Read the model definition and answer for the solid it produces. Units are mm, in the model's axes. Give positions to 0.01 mm unless a question says otherwise; leave off trailing zeros. Loops run counter-clockwise (first coordinate to the right, second up) from the corner with the lowest first, then second, coordinate; pieces in that order, holes last. Notation, with made-up numbers: (-32, -15) - (15, -15) arc R11 ccw to (15, 3) - close; hole circle Ø4 at (-8, 41). An arc over 180 degrees is marked (long way). Write item = value, one per line.
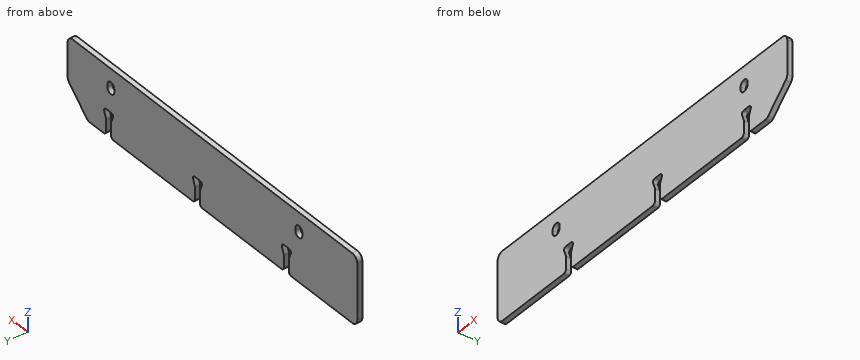
```python
from build123d import *

# Parameters (mm, degrees)
SKETCH2_W           = 114
SKETCH2_H           = 21.5
BOSS_EXTRUDE1_DEPTH = 1.5875
CHAMFER1_SIZE       = 8
FILLET1_R           = 2
CUT_EXTRUDE1_DEPTH  = 2.5875
LPATTERN1_COUNT     = 3
LPATTERN1_PITCH     = 35
FILLET2_R           = 1
FILLET3_R           = 1


with BuildPart() as part:
    # Sketch2 → Boss-Extrude1 (new body)
    with BuildSketch(Plane(origin=(0, 0, 0), x_dir=(1, 0, 0), z_dir=(0, 1, 0))):
        with Locations((-3, 10.75)):
            Rectangle(SKETCH2_W, SKETCH2_H)
        with BuildLine():
            Line((-38.35, 5.5), (-38.35, 6.5))
            ThreePointArc((-38.35, 6.5), (-37, 7.85), (-35.65, 6.5))
            Line((-35.65, 6.5), (-35.65, 5.5))
            ThreePointArc((-35.65, 5.5), (-37, 4.15), (-38.35, 5.5))
        make_face(mode=Mode.SUBTRACT)
        with BuildLine():
            Line((35.65, 5.5), (35.65, 6.5))
            ThreePointArc((35.65, 6.5), (37, 7.85), (38.35, 6.5))
            Line((38.35, 6.5), (38.35, 5.5))
            ThreePointArc((38.35, 5.5), (37, 4.15), (35.65, 5.5))
        make_face(mode=Mode.SUBTRACT)
    extrude(amount=BOSS_EXTRUDE1_DEPTH)

    # Chamfer1
    chamfer1_edges = [part.edges().sort_by_distance(p)[0] for p in [
        (54, 0.79375, -21.5),
    ]]
    chamfer(chamfer1_edges, length=CHAMFER1_SIZE)

    # Fillet1
    fillet1_edges = [part.edges().sort_by_distance(p)[0] for p in [
        (46, 0.79375, -21.5),
        (54, 0.79375, -13.5),
        (-60, 0.79375, 0),
        (-60, 0.79375, -21.5),
        (54, 0.79375, 0),
    ]]
    fillet(fillet1_edges, radius=FILLET1_R)

    # Sketch3 → Cut-Extrude1 (cut, through all)
    with BuildSketch(Plane(origin=(0, 0, 0), x_dir=(1, 0, 0), z_dir=(0, 1, 0))):
        with BuildLine():
            Line((-33.075, 21.5), (-31.125, 21.5))
            Line((-31.125, 21.5), (-31.125, 16.63904352))
            Line((-31.125, 16.63904352), (-30.373245903, 14.573616115))
            ThreePointArc((-30.373245903, 14.573616115), (-30.469678365, 13.841138851), (-31.125, 13.5))
            Line((-31.125, 13.5), (-33.075, 13.5))
            ThreePointArc((-33.075, 13.5), (-33.730321635, 13.841138851), (-33.826754097, 14.573616115))
            Line((-33.826754097, 14.573616115), (-33.075, 16.63904352))
            Line((-33.075, 16.63904352), (-33.075, 21.5))
        make_face()
    cut_extrude1 = extrude(amount=CUT_EXTRUDE1_DEPTH, mode=Mode.SUBTRACT)

    # LPattern1: Cut-Extrude1 ×3
    with Locations(*[(i * LPATTERN1_PITCH, 0, 0) for i in range(1, LPATTERN1_COUNT)]):
        add(cut_extrude1, mode=Mode.SUBTRACT)

    # Fillet2
    fillet2_edges = [part.edges().sort_by_distance(p)[0] for p in [
        (3.875, 0.79375, -21.5),
        (1.925, 0.79375, -21.5),
        (38.875, 0.79375, -21.5),
        (36.925, 0.79375, -21.5),
        (-33.075, 0.79375, -21.5),
        (-31.125, 0.79375, -21.5),
    ]]
    fillet(fillet2_edges, radius=FILLET2_R)

    # Fillet3
    fillet3_edges = [part.edges().sort_by_distance(p)[0] for p in [
        (1.925, 0.79375, -16.63904352),
        (3.875, 0.79375, -16.63904352),
        (36.925, 0.79375, -16.63904352),
        (38.875, 0.79375, -16.63904352),
        (-33.075, 0.79375, -16.63904352),
        (-31.125, 0.79375, -16.63904352),
    ]]
    fillet(fillet3_edges, radius=FILLET3_R)


solid = part.part
```
1) Find the intervals of material crossed by probe 1 along X at (y, z) = (0.95, -5.5); probe 2 along X at (y, z) = (0.35, -14); probe 3 along X at (y, z) = (0.2, -7.25), in increasing order.
Output:
probe_1 = -60 to -38.35, -35.65 to 35.65, 38.35 to 54
probe_2 = -60 to -33.82, -30.38 to 1.18, 4.62 to 36.18, 39.62 to 53.5
probe_3 = -60 to -38.12, -35.88 to 35.88, 38.12 to 54
2) A cutting plane is placed at A-A on x = -37. Determine the outline of the cut face in (y, z), then the cut area to 3 significant figures.
Output:
outline = (0, -21.5) - (1.59, -21.5) - (1.59, -7.85) - (0, -7.85) - close; (0, -4.15) - (1.59, -4.15) - (1.59, 0) - (0, 0) - close
area = 28.3 mm²
3) A cutting plane is placed at B-B on y = 1.05. Give the number of separate pieces and of enclosed holes in the cut face, then the cut area to 3 significant figures.
Output:
separate_pieces = 1
enclosed_holes = 2
area = 2,340 mm²
4) Each of these flat-tipped pins is pushed along its axis until it touches: P1, Ø0.5, axis at x = 38, y = 1, coming from the -Z side; P2, Ø0.8, axis at y = 0.5, z = -18, coming from the +X side. Where does it stop, or does it pass through?
Output:
P1 = -13.5
P2 = 49.9
